from build123d import *

# Parameters (mm, degrees)
ESQUISSE1_R        = 7.5
ESQUISSE1_R_2      = 4
BOSS_EXTRU_1_DEPTH = 12
CHANFREIN1_SIZE    = 0.2


with BuildPart() as part:
    # Esquisse1 → Boss.-Extru.1 (new, symmetric)
    with BuildSketch(Plane.XY):
        Circle(ESQUISSE1_R)
        Circle(ESQUISSE1_R_2, mode=Mode.SUBTRACT)
    extrude(amount=BOSS_EXTRU_1_DEPTH, both=True)

    # Chanfrein1
    chanfrein1_edges = [part.edges().sort_by_distance(p)[0] for p in [
        (-7.5, 0, -12),
        (-7.5, 0, 12),
        (-4, 0, -12),
        (-4, 0, 12),
    ]]
    chamfer(chanfrein1_edges, length=CHANFREIN1_SIZE)

    # Esquisse2 → Enlèvement de matière-Révolution1 (revolve, cut)
    with BuildSketch(Plane(origin=(0, 0, 0), x_dir=(0, 0, -1), z_dir=(1, 0, 0)), mode=Mode.PRIVATE) as enl_vement_de_mati_re_r_volution1_sk:
        with BuildLine():
            Line((-9, 7.5), (-8, 7.5))
            ThreePointArc((-8, 7.5), (-8.5, 7), (-9, 7.5))
        make_face()
    enl_vement_de_mati_re_r_volution1 = revolve(enl_vement_de_mati_re_r_volution1_sk.sketch.rotate(Axis((0, 0, 55), (0, 0, -1)), 90), axis=Axis((0, 0, 55), (0, 0, -1)), mode=Mode.SUBTRACT)

    # Symétrie1: Enlèvement de matière-Révolution1 across plane
    add(enl_vement_de_mati_re_r_volution1.mirror(Plane.XY), mode=Mode.SUBTRACT)


solid = part.part
Can you work these out from the model? Positions are in its coordinate system, mm. Give positions to 0.01 mm unless a question says otherwise; leave off trailing zeros. Loops run counter-clockwise (first coordinate to the right, second up) from the corner with the lowest first, then second, coordinate; pieces in that order, holes last. Notation, with made-up numbers: (-37.75, 10) - (-16.75, 10) arc R19 ccw to (-16.75, 34) - close; hole circle Ø3 at (-6, -12). An arc over 180 degrees is marked (long way). One line per item, written item: value.
(1) I need wall thicknesses on line 1 along Y through (x, z) = (0, 1.75); line 2 along Y through (x, z) = (3, 6.5); line 3 along X through (y, z) = (1.25, -10.25). Which ranges of each line are inside material? Lowest first, please.
Verdict:
line 1: -7.5 to -4, 4 to 7.5
line 2: -6.87 to -2.65, 2.65 to 6.87
line 3: -7.4 to -3.8, 3.8 to 7.4
(2) If we section it at A-A, the plane y = 0: List the corners of the cut face in (x, z) for me.
Verdict:
outline: (-7.5, -11.8) - (-7.3, -12) - (-4.2, -12) - (-4, -11.8) - (-4, 11.8) - (-4.2, 12) - (-7.3, 12) - (-7.5, 11.8) - (-7.5, 9) arc R0.5 cw to (-7.5, 8) - (-7.5, -8) arc R0.5 cw to (-7.5, -9) - close; (4, -11.8) - (4.2, -12) - (7.3, -12) - (7.5, -11.8) - (7.5, -9) arc R0.5 cw to (7.5, -8) - (7.5, 8) arc R0.5 cw to (7.5, 9) - (7.5, 11.8) - (7.3, 12) - (4.2, 12) - (4, 11.8) - close
(3) If we mould it in two halves opening along Y, with no side actions, what happens to faces 1 (the face through (-7.493, 0.33, -10.38)), 2 (the face through (-0.867, -3.905, -0.165)), 3 (the face through (3.1, -3.1, -12))? For each: released by +Y, released by -Y, zero draft, split by the parting line, or undercut.
Verdict:
face 1: split by the parting line
face 2: undercut
face 3: zero draft
(4) I'm going to push flat-ended pins straight in: pin 1 (3 mm diameter, centred on x = 5.5, z = -8, fed in from +Y); pin 2 (6 mm diameter, centred on x = 1.5, y = -3.5, fed in from +Z); pin 3 (2 mm diameter, centred on x = -4.5, z = -1, fed in from -Y); pin 4 (6 mm diameter, centred on y = 5, z = 8, fed in from -X). Where does each tip first touch, or does it pass through?
Verdict:
pin 1: y = 6.34
pin 2: z = 12
pin 3: y = -6.63
pin 4: x = -7.23
(5) If we section it at C-C, the plane z = 0.5: List the corners of the cut face in (x, y) for me, plus the area to 3 significant figures.
Verdict:
outline: circle Ø15 at (0, 0); hole circle Ø8 at (0, 0)
area: 126 mm^2
